Study the drawing (mm; zero at the part's minimum x, y, z) and answer. A direction names the side the tool comes from. Coordinates: 2 decimals unless noted, no trailing zeros. Loops run counter-clockwise (first coordinate to the right, second up) from the corner with the lowest first, then second, coordinate; pieces in that order, holes last.
Q1. Section B-B (x = 3.75) is taken. Give the vertices of the cut face in (y, z).
Q2. Straight lines are drawn through the part: line 1 (Z direction, x = 7.85, y = 11.5); line 2 (Y direction, x = 8.35, z = 15.5); line 3 (Z direction, x = 8.75, y = 4.5) (1 decimal). For each, find the intervals that lie inside material, in ascending order.
Q3. Section C-C (z = 11.5) is taken. Give the vertices of the cut face in (x, y), then the cut area to 3 significant figures.
Q4. Flat-ended cylindrical pins translate along their axes: P1, Ø3, axis at x = 2, z = 15.5, coming from the -Y side; P2, Ø2, axis at x = 3.5, y = 11, coming from the +Z side; P3, Ø1.5, axis at y = 14, z = 17, coming from the -X side. Find the tip coordinate at first contact, or state that the pin passes through.
Q5. Section D-D (x = 5.5) is taken. Give the vertices of the cut face in (y, z), then the cut area to 3 significant figures.
Q6. Which of the six approach directions +Z, -Z, +X, -X, +Y, -Y give full straight-line access (tool end or side, diameter ignored) to the marked faces 4, 5 and 6?
Q7. The mould has two halves that part along Z. Classify the marked faces 1, 2 and 3: pulls with the +Z half, pulls with the -Z half, needs draft (parallel to the pull), parting line crosses it, or undercut.
Q8. Section A-A (y = 11.5) is taken. Give the vertices of the cut face in (x, z), then the cut area to 3 significant figures.
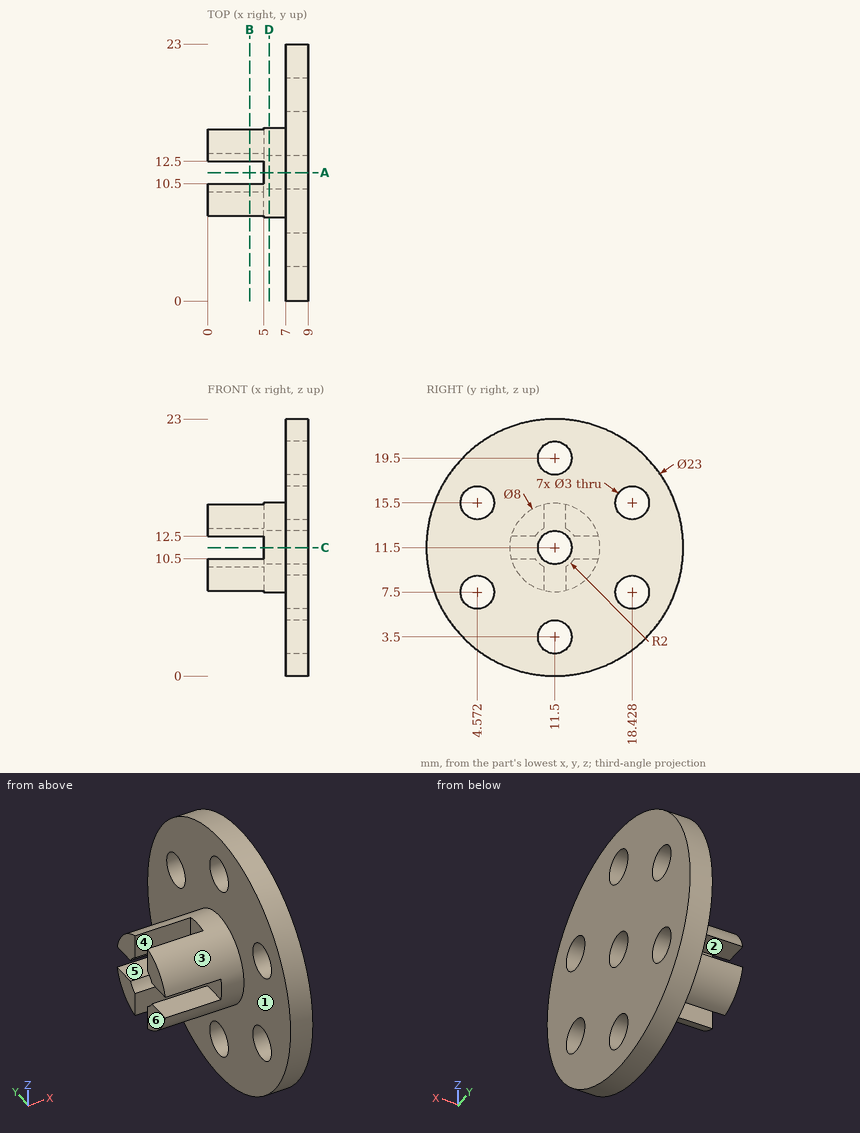
Numbers:
1. outline: (7.63, 10.5) arc R4 ccw to (10.5, 7.63) - (10.5, 9.77) arc R2 cw to (9.77, 10.5) - close; (7.63, 12.5) - (9.77, 12.5) arc R2 cw to (10.5, 13.23) - (10.5, 15.37) arc R4 ccw to start; (12.5, 7.63) arc R4 ccw to (15.37, 10.5) - (13.23, 10.5) arc R2 cw to (12.5, 9.77) - close; (12.5, 13.23) arc R2 cw to (13.23, 12.5) - (15.37, 12.5) arc R4 ccw to (12.5, 15.37) - close
2. line 1: z = 0 to 2, 5 to 10, 13 to 18, 21 to 23
2. line 2: y = 0.72 to 3.07, 6.07 to 16.93, 19.93 to 22.28
2. line 3: z = 2.4 to 6, 9 to 14, 17 to 20.6
3. outline: (5, 7.5) - (7, 7.5) - (7, 0) - (9, 0) - (9, 10) - (5, 10) - close; (5, 13) - (9, 13) - (9, 23) - (7, 23) - (7, 15.5) - (5, 15.5) - close
3. area: 50.0 mm2
4. P1: stops at y = 8.38
4. P2: stops at z = 15.37
4. P3: stops at x = 7
5. outline: circle Ø8 at (11.5, 11.5); hole circle Ø3 at (11.5, 11.5)
5. area: 43.2 mm2
6. face 4: +Z, -Z, -X
6. face 5: -X, +Y, -Y
6. face 6: +Z, -Z, -X, +Y, -Y
7. face 1: needs draft
7. face 2: undercut
7. face 3: parting line crosses it
8. outline: (5, 7.5) - (7, 7.5) - (7, 5) - (9, 5) - (9, 10) - (5, 10) - close; (5, 13) - (9, 13) - (9, 18) - (7, 18) - (7, 15.5) - (5, 15.5) - close; (7, 0) - (9, 0) - (9, 2) - (7, 2) - close; (7, 21) - (9, 21) - (9, 23) - (7, 23) - close
8. area: 38.0 mm2
